Read the model definition and answer for the solid it produces. Units are mm, in the model's axes. A direction names the side the tool comes from. Coordinates: 2 decimals unless noted, no trailing zeros. Loops run counter-clockwise (first coordinate to the right, second up) from the corner with the lowest first, then second, coordinate; pieces in that order, holes last. Notation, with made-up numbers: (9, 86.25) -> (22, 86.25) arc R22 cw to (22, 96.25) -> close; hole circle Ø8 at (-9.75, 59.25). An arc over 180 degrees is marked (long way). Answer in a Markdown table with one row per item.
```python
from build123d import *

# Parameters (mm, degrees)
SKETCH1_R           = 10.5
SKETCH1_R_2         = 0.8
BOSS_EXTRUDE1_DEPTH = 2
SKETCH2_R           = 1.5
CUT_EXTRUDE1_DEPTH  = 2
SKETCH2_3_R         = 4.22
SKETCH2_3_R_2       = 2.72
BOSS_EXTRUDE2_DEPTH = 3.4


with BuildPart() as part:
    # Sketch1 → Boss-Extrude1 (new body)
    with BuildSketch(Plane(origin=(0, 0, 0), x_dir=(1, 0, 0), z_dir=(0, 1, 0))):
        with Locations(Location((0, 0, 0), (0, 0, 270))):
            Circle(SKETCH1_R)
        with Locations(Location((0, 7.2, 0), (0, 0, 270))):
            Circle(SKETCH1_R_2, mode=Mode.SUBTRACT)
        with Locations(Location((7.2, 0, 0), (0, 0, 270))):
            Circle(SKETCH1_R_2, mode=Mode.SUBTRACT)
        with Locations(Location((0, -7.2, 0), (0, 0, 270))):
            Circle(SKETCH1_R_2, mode=Mode.SUBTRACT)
        with Locations(Location((-7.2, 0, 0), (0, 0, 270))):
            Circle(SKETCH1_R_2, mode=Mode.SUBTRACT)
    extrude(amount=BOSS_EXTRUDE1_DEPTH)

    # Sketch2 → Cut-Extrude1 (cut)
    with BuildSketch(Plane(origin=(0, 2, 0), x_dir=(1, 0, 0), z_dir=(0, 1, 0))):
        with Locations(Location((0, 0, 0), (0, 0, 270))):
            Circle(SKETCH2_R)
    extrude(amount=-CUT_EXTRUDE1_DEPTH, mode=Mode.SUBTRACT)

    # Sketch2_3 → Boss-Extrude2 (add)
    with BuildSketch(Plane(origin=(0, 2, 0), x_dir=(1, 0, 0), z_dir=(0, 1, 0))):
        with Locations(Location((0, 0, 0), (0, 0, 270))):
            Circle(SKETCH2_3_R)
        with Locations(Location((0, 0, 0), (0, 0, 270))):
            Circle(SKETCH2_3_R_2, mode=Mode.SUBTRACT)
    extrude(amount=BOSS_EXTRUDE2_DEPTH)


solid = part.part
```
1. A tool of negligible diameter and unlimited length cuts with its end or side. For faces 4 (the cylindrical face through (-6.407, 0.986, -0.104)), 5 (the flat face through (-1.2, 2, 1.2)), from which of +Z, -Z, +X, -X, +Y, -Y can it reach the whole face along a straight path? Write none if from no direction.
A:
| item | result |
|---|---|
| face 4 | +Y, -Y |
| face 5 | +Y |
2. Find the intervals of material crossed by probe 1 along X at (y, z) = (1.5, 0); probe 2 along X at (y, z) = (3.05, 0); probe 3 along Y at (x, z) = (7.5, 1.5), in increasing order.
A:
| item | result |
|---|---|
| probe 1 | x = -10.5 to -8, -6.4 to -1.5, 1.5 to 6.4, 8 to 10.5 |
| probe 2 | x = -4.22 to -2.72, 2.72 to 4.22 |
| probe 3 | y = 0 to 2 |
3. Given pin 1 Ø10 at (x, z) = (-4.5, -5) entering from +Y; pin 2 Ø1.5 at (y, z) = (1.5, -1.5) entering from +X; pin 3 Ø1.8 at (x, z) = (0, 7.2) entering from +Y; pin 4 Ø1 at (x, z) = (7.2, 0) entering from -Y, each flat-ended and moving along its own axis, determine where each tip first touches the part or whether it passes through.
A:
| item | result |
|---|---|
| pin 1 | stops at y = 5.4 |
| pin 2 | stops at x = 10.47 |
| pin 3 | stops at y = 2 |
| pin 4 | passes through |
4. A cutting plane is placed at A-A on x = 0. Give the vertices of the cut face in (y, z).
A:
| item | result |
|---|---|
| outline | (0, -10.5) -> (2, -10.5) -> (2, -8) -> (0, -8) -> close; (0, -6.4) -> (2, -6.4) -> (2, -4.22) -> (5.4, -4.22) -> (5.4, -2.72) -> (2, -2.72) -> (2, -1.5) -> (0, -1.5) -> close; (0, 1.5) -> (2, 1.5) -> (2, 2.72) -> (5.4, 2.72) -> (5.4, 4.22) -> (2, 4.22) -> (2, 6.4) -> (0, 6.4) -> close; (0, 8) -> (2, 8) -> (2, 10.5) -> (0, 10.5) -> close |
5. A cutting plane is placed at B-B on z = 0. Give the vertices of the cut face in (x, y).
A:
| item | result |
|---|---|
| outline | (-10.5, 0) -> (-8, 0) -> (-8, 2) -> (-10.5, 2) -> close; (-6.4, 0) -> (-1.5, 0) -> (-1.5, 2) -> (-2.72, 2) -> (-2.72, 5.4) -> (-4.22, 5.4) -> (-4.22, 2) -> (-6.4, 2) -> close; (1.5, 0) -> (6.4, 0) -> (6.4, 2) -> (4.22, 2) -> (4.22, 5.4) -> (2.72, 5.4) -> (2.72, 2) -> (1.5, 2) -> close; (8, 0) -> (10.5, 0) -> (10.5, 2) -> (8, 2) -> close |
6. The mould has two halves that part along X. Classify faces 1 (the cylindrical face through (8, 1, 0)), 2 (the cylindrical face through (4.184, 3.676, -0.549)), 3 (the flat face through (-3, 5.4, 0)): pulls with the +X half, pulls with the -X half, needs draft (parallel to the pull), parting line crosses it, or undercut.
A:
| item | result |
|---|---|
| face 1 | undercut |
| face 2 | parting line crosses it |
| face 3 | needs draft |
7. A cutting plane is placed at D-D on y = 3.7. Give the vertices of the cut face in (x, z).
A:
| item | result |
|---|---|
| outline | circle Ø8.44 at (0, 0); hole circle Ø5.44 at (0, 0) |
8. A cutting plane is placed at C-C on x = 7.2. Give the vertices of the cut face in (y, z).
A:
| item | result |
|---|---|
| outline | (0, -7.64) -> (2, -7.64) -> (2, -0.8) -> (0, -0.8) -> close; (0, 0.8) -> (2, 0.8) -> (2, 7.64) -> (0, 7.64) -> close |
